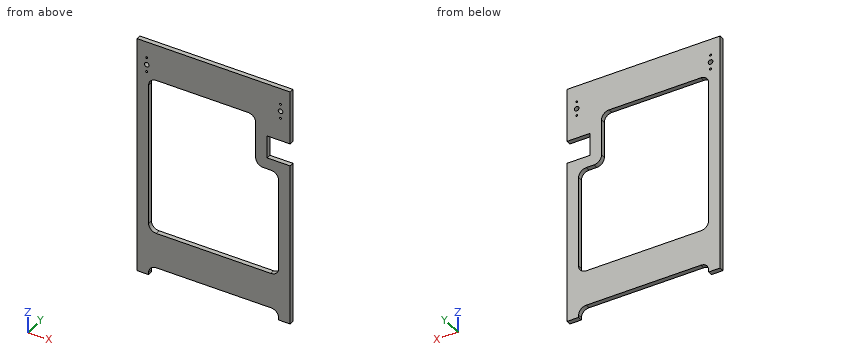
```python
from build123d import *

# Parameters (mm, degrees)
F1_R     = 2.5
F1_R_2   = 6
F1_W     = 400
F1_H     = 12
F1_H_2   = 60
F2_DEPTH = 12


with BuildPart() as f2:
    # F1 (on Front) → F2 (new body)
    with BuildSketch(Plane.XZ):
        Polygon((200, 232), (200, 374), (-200, 374), (-200, -150), (200, -150), (200, 172), (140, 172), (140, 232), align=None)
        with Locations((-175, 293)):
            Circle(F1_R, mode=Mode.SUBTRACT)
        with Locations((-175, 312)):
            Circle(F1_R_2, mode=Mode.SUBTRACT)
        with Locations((-175, 331)):
            Circle(F1_R, mode=Mode.SUBTRACT)
        with BuildLine():
            Line((-150, 278), (90, 278))
            ThreePointArc((90, 278), (104.1421356237, 272.1421356237), (110, 258))
            Line((110, 258), (110, 162))
            ThreePointArc((110, 162), (115.8578643763, 147.8578643763), (130, 142))
            Line((130, 142), (150, 142))
            ThreePointArc((150, 142), (164.1421356237, 136.1421356237), (170, 122))
            Line((170, 122), (170, -120))
            ThreePointArc((170, -120), (164.1421356237, -134.1421356237), (150, -140))
            Line((150, -140), (-150, -140))
            ThreePointArc((-150, -140), (-164.1421356237, -134.1421356237), (-170, -120))
            Line((-170, -120), (-170, 258))
            ThreePointArc((-170, 258), (-164.1421356237, 272.1421356237), (-150, 278))
        make_face(mode=Mode.SUBTRACT)
        with Locations((175, 293)):
            Circle(F1_R, mode=Mode.SUBTRACT)
        with Locations((175, 312)):
            Circle(F1_R_2, mode=Mode.SUBTRACT)
        with Locations((175, 331)):
            Circle(F1_R, mode=Mode.SUBTRACT)
        with Locations((0, -156)):
            Rectangle(F1_W, F1_H)
        with Locations((0, -192)):
            Rectangle(F1_W, F1_H_2)
        Polygon((200, -222), (-200, -222), (-200, -234), (-150, -234), (150, -234), (200, -234), align=None)
        with BuildLine():
            Line((200, -260), (200, -234))
            Line((200, -234), (150, -234))
            ThreePointArc((150, -234), (164.1421356237, -239.8578643763), (170, -254))
            Line((170, -254), (170, -260))
            Line((170, -260), (200, -260))
        make_face()
        with BuildLine():
            Line((-150, -234), (-200, -234))
            Line((-200, -234), (-200, -260))
            Line((-200, -260), (-170, -260))
            Line((-170, -260), (-170, -254))
            ThreePointArc((-170, -254), (-164.1421356237, -239.8578643763), (-150, -234))
        make_face()
    extrude(amount=F2_DEPTH)


solid = f2.part
```
Here's how the part is built. I have some questions about the finished solid (model axes, mm). Round coordinates to 2 decimals unless told otherwise and drop trailing zeros. Write each loop counter-clockwise with the first axis right and the second up, starting at its lowest first coordinate (ties: lowest second). Pieces come first, ordered by that corner, then holes.
Q1. If we section it at C-C on y = -3.75: Give the number of separate pieces and of enclosed holes in the cut face, plus the area to 3 significant figures.
Q2. Will this pin go through, and if not, where does the flat tip stop? P1, Ø6, axis at x = -20.5, y = -8.5, coming from the -Z side.
Q3. Please list where these lines run through material, in increasing order: probe 1 along X at (y, z) = (-9.25, 331); probe 2 along Z at (x, y) = (148, -1); probe 3 along X at (y, z) = (-4.75, 312).
Q4. If we section it at B-B on x = -114: Write out the boundary of the cut face in (y, z), plus the area to 3 significant figures.
Q5. If we section it at A-A on z = 23.5: Write out the boundary of the cut face in (x, y).
Answer below:
1. separate pieces: 1
1. enclosed holes: 7
1. area: 107,000 mm2
2. P1: stops at z = -234
3. probe 1: x = -200 to -177.5, -172.5 to 172.5, 177.5 to 200
3. probe 2: z = -234 to -140, 142 to 172, 232 to 374
3. probe 3: x = -200 to -181, -169 to 169, 181 to 200
4. outline: (-12, -234) - (0, -234) - (0, -140) - (-12, -140) - close; (-12, 278) - (0, 278) - (0, 374) - (-12, 374) - close
4. area: 2,280 mm2
5. outline: (-200, -12) - (-170, -12) - (-170, 0) - (-200, 0) - close; (170, -12) - (200, -12) - (200, 0) - (170, 0) - close
